Part model, mm, in its own coordinate system. Face numbers are marked on the shaded views. A direction names the side the tool comes from. Give positions to 0.01 mm unless a question says otherwise; leave off trailing zeros. Write each loop counter-clockwise with the first axis right and the second up, starting at its lowest first coordinate (ties: lowest second). Pieces come first, ordered by that corner, then holes. Notation, with made-up numbers: M 47.5,-22 L 57.5,-22 A35 ccw 57.5,12 Z; hole C 59,56 d6. An arc over 180 degrees is marked long. Use a Markdown table: item, result.
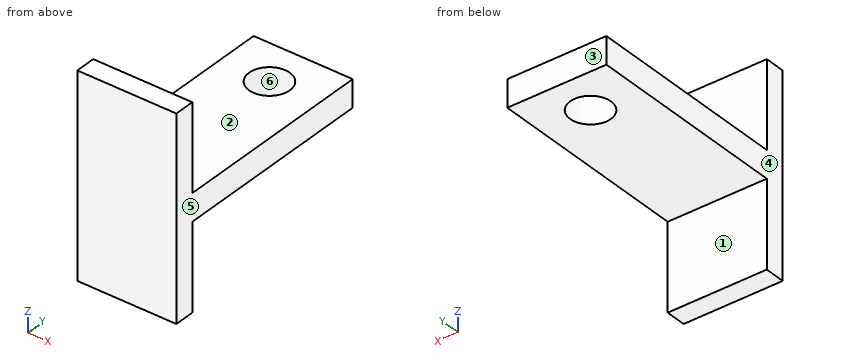
```python
from build123d import *

# Parameters (mm, degrees)
BOSS_EXTRUDE1_DEPTH = 3.65125
SKETCH3_R           = 1.5
CUT_EXTRUDE1_DEPTH  = 19.94850642


with BuildPart() as part:
    # Sketch1 → Boss-Extrude1 (new, symmetric)
    with BuildSketch(Plane(origin=(0, 0, 0), x_dir=(0, 0, -1), z_dir=(1, 0, 0))):
        Polygon((-7.35, 0), (7.35, 0), (7.35, 1.5), (1, 1.5), (1, 16.613), (-1, 16.613), (-1, 1.5), (-7.35, 1.5), align=None)
    extrude(amount=BOSS_EXTRUDE1_DEPTH, both=True)

    # Sketch3 → Cut-Extrude1 (cut, through all)
    with BuildSketch(Plane.XY.offset(1)):
        with Locations((0, 13.438)):
            Circle(SKETCH3_R)
    extrude(amount=-CUT_EXTRUDE1_DEPTH, mode=Mode.SUBTRACT)


solid = part.part
```
1. Cut at A-A, the plane x = 0. Give the cut face in (y, z).
Findings below:
| item | result |
|---|---|
| outline | M 0,-7.35 L 1.5,-7.35 L 1.5,-1 L 11.94,-1 L 11.94,1 L 1.5,1 L 1.5,7.35 L 0,7.35 Z; M 14.94,-1 L 16.61,-1 L 16.61,1 L 14.94,1 Z |
2. Drop flat-ended pins along their axis: P1, Ø2, axis at x = 0.5, y = 7.5, coming from the -Z side; P2, Ø6, axis at y = 11.5, z = 5.5, coming from the +X side; P3, Ø2, axis at x = 1.5, z = 6, coming from the +Y side. Give the stop position or say it passes through.
Findings below:
| item | result |
|---|---|
| P1 | z = -1 |
| P2 | through |
| P3 | y = 1.5 |
3. Cut at B-B, the plane x = 3.25. Give the cut face in (y, z).
Findings below:
| item | result |
|---|---|
| outline | M 0,-7.35 L 1.5,-7.35 L 1.5,-1 L 16.61,-1 L 16.61,1 L 1.5,1 L 1.5,7.35 L 0,7.35 Z |
4. Two-plate mould, pull along X, no slides. Class the marked faces 4, 5 and 6: released by +X, released by -X, zero draft, split by the parting line, or undercut.
Findings below:
| item | result |
|---|---|
| face 4 | released by -X |
| face 5 | released by +X |
| face 6 | undercut |
5. Drill centre lines: L1, parallel to Y at x = 0, z = -0.1; L2, parallel to Z at x = 1, y = 8; L3, parallel to Y at x = -1, z = 4.75. Where is each one in solid material? Low to high.
Findings below:
| item | result |
|---|---|
| L1 | 0 to 11.94, 14.94 to 16.61 |
| L2 | -1 to 1 |
| L3 | 0 to 1.5 |
6. Tool access for the marked faces 1, 2 and 3: list every direction of +Z, -Z, +X, -X, +Y, -Y with a clear straight run to the whole face (end or side of a thin tool).
Findings below:
| item | result |
|---|---|
| face 1 | -Z, +X, -X, +Y |
| face 2 | +Z, +X, -X, +Y |
| face 3 | +Z, -Z, +X, -X, +Y |
7. Cut at D-D, the plane z = 5.75. Give the cut face in (x, y).
Findings below:
| item | result |
|---|---|
| outline | M -3.65,0 L 3.65,0 L 3.65,1.5 L -3.65,1.5 Z |
8. Cut at C-C, the plane y = 4.5. Give the cut face in (x, z), then the cut area to 3 significant figures.
Findings below:
| item | result |
|---|---|
| outline | M -3.65,-1 L 3.65,-1 L 3.65,1 L -3.65,1 Z |
| area | 14.6 mm2 |
